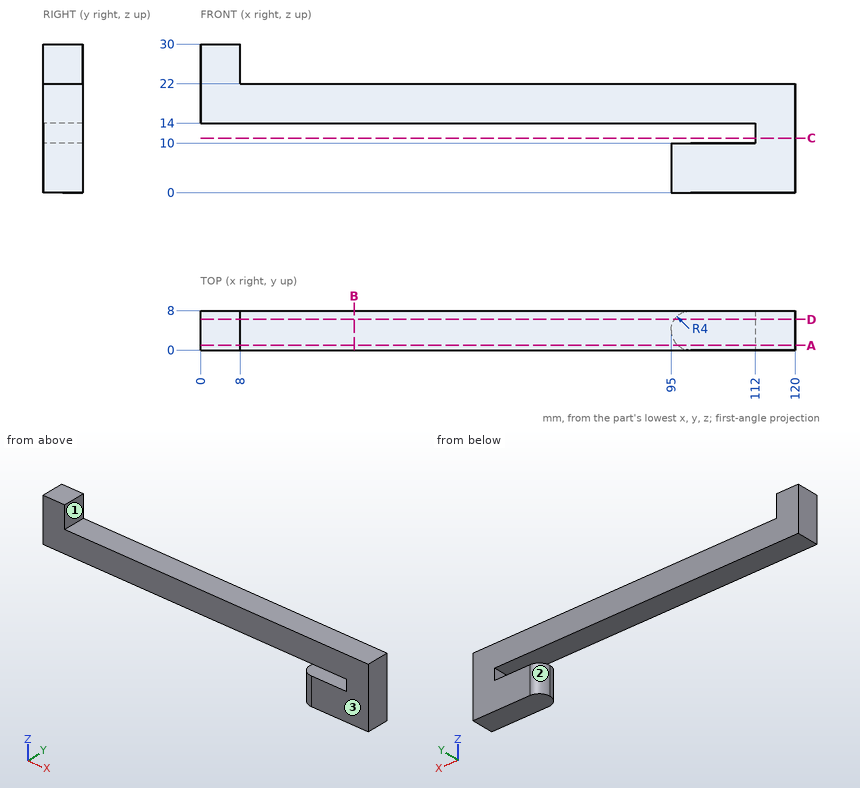
For this review, use the dimensioned drawing (mm, ordinates from the lowest corner) and the shaded views. A direction names the side the tool comes from. Round coordinates to 2 decimals unless told otherwise and drop trailing zeros. Write each loop counter-clockwise with the first axis right and the second up, starting at its lowest first coordinate (ties: lowest second). Pieces come first, ordered by that corner, then holes. Notation, with made-up numbers: M 42.25,41 L 61.25,41 A17 cw 61.25,45 Z; hole C 63,5.25 d11. An arc over 180 degrees is marked long. Answer as CSV lines item,"result". Start each with the question number.
Q1. Wall thickness on line 1 along Z through (x, y) = (101, 7.25); line 2 along Z through (x, y) = (52, 7.5); line 3 along X through (y, z) = (1.25, 12): over which ranges is each line inside the solid? List them lowest first.
Q2. Clearance check with flat-ended pins moving along their axes: P1, Ø2.5, axis at y = 3, z = 27, coming from the +X side; P2, Ø2.5, axis at x = 87.5, y = 5.5, coming from the +Z side; P3, Ø1.5, axis at x = 54, y = 4.5, coming from the -Z side. State where each tip first meets the part, or that it passes through.
Q3. Consider section A-A, the plane y = 1. Give the boundary of the cut face in (x, z), then the cut area to 3 significant figures.
Q4. Tool access review of the marked faces 1, 2 and 3: name each direction out of +Z, -Z, +X, -X, +Y, -Y from which nothing blocks a thin tool from reaching the whole face with its end or side.
Q5. Consider section D-D, the plane y = 6.25. Give the boundary of the cut face in (x, z).
Q6. Consider section B-B, the plane x = 31. Give the boundary of the cut face in (y, z), then the cut area to 3 significant figures.
Q7. Consider section C-C, the plane z = 11. Give the boundary of the cut face in (x, y).
Result set:
1,line 1,"z = 0 to 10, 14 to 22"
1,line 2,"z = 14 to 22"
1,line 3,"x = 112 to 120"
2,P1,"stops at x = 8"
2,P2,"stops at z = 22"
2,P3,"stops at z = 14"
3,outline,"M 0,14 L 112,14 L 112,10 L 96.35,10 L 96.35,0 L 120,0 L 120,22 L 8,22 L 8,30 L 0,30 Z"
3,area,"1,290 mm²"
4,face 1,"+Z, +X, +Y, -Y"
4,face 2,"-Z, -X, +Y"
4,face 3,"+Z, -Z, +X, -X, -Y"
5,outline,"M 0,14 L 112,14 L 112,10 L 95.69,10 L 95.69,0 L 120,0 L 120,22 L 8,22 L 8,30 L 0,30 Z"
6,outline,"M 0,14 L 8,14 L 8,22 L 0,22 Z"
6,area,"64.0 mm²"
7,outline,"M 112,0 L 120,0 L 120,8 L 112,8 Z"
